The listing builds one solid part. Answer for the finished solid, in the listing's coordinates (mm). Coordinates: 2 decimals unless noted, no trailing zeros. Write each loop counter-clockwise with the first axis right and the second up, starting at its lowest first coordinate (ties: lowest second). Pieces come first, ordered by that corner, then holes.
(1) For a pull along Y with two mould halves and no side action, classify faces 1 (the flat face through (0, -10, 0)), 2 (the flat face through (0, 21, 2)), 3 (the cylindrical face through (-17, 15.57, 1.97)) as +Y half, -Y half, draft (parallel to the pull), parting line (faces both ways), or undercut.
(2) The part is cut by section C-C on x = 15.5. Determine the outline of the cut face in (y, z), plus the area to 3 significant figures.
(3) Straight lines are drawn through the part: line 1 (Y direction, x = -15.5, z = 2.85); line 2 (Y direction, x = 11, z = 1.2); line 3 (X direction, y = -32, z = 0.7). For each, find the intervals that lie inside material, in ascending order.
(4) The part is cut by section D-D on y = 0. Determine the outline of the cut face in (x, z), plus the area to 3 significant figures.
(5) The part is cut by section B-B on x = 0. Determine the outline of the cut face in (y, z).
(6) The part is cut by section A-A on y = -31. Determine the outline of the cut face in (x, z), plus the area to 3 significant figures.
from build123d import *

# Parameters (mm, degrees)
SKETCH1_W           = 42
SKETCH1_H           = 42
SKETCH1_R           = 4
SKETCH1_R_2         = 1.5
BOSS_EXTRUDE1_DEPTH = 4
SKETCH3_W           = 42
SKETCH3_H           = 4
BOSS_EXTRUDE2_DEPTH = 20
SKETCH4_R           = 2.5
CUT_EXTRUDE2_DEPTH  = 20


with BuildPart() as part:
    # Sketch1 → Boss-Extrude1 (new body)
    with BuildSketch(Plane.XY):
        Rectangle(SKETCH1_W, SKETCH1_H)
        Circle(SKETCH1_R, mode=Mode.SUBTRACT)
        with Locations((-15.5, 15.5)):
            Circle(SKETCH1_R_2, mode=Mode.SUBTRACT)
        with Locations((15.5, 15.5)):
            Circle(SKETCH1_R_2, mode=Mode.SUBTRACT)
        with Locations((15.5, -15.5)):
            Circle(SKETCH1_R_2, mode=Mode.SUBTRACT)
        with Locations((-15.5, -15.5)):
            Circle(SKETCH1_R_2, mode=Mode.SUBTRACT)
    extrude(amount=BOSS_EXTRUDE1_DEPTH)

    # Sketch3 → Boss-Extrude2 (add)
    with BuildSketch(Plane.XZ.offset(21)):
        with Locations((0, 2)):
            Rectangle(SKETCH3_W, SKETCH3_H)
    extrude(amount=BOSS_EXTRUDE2_DEPTH)

    # Sketch4 → Cut-Extrude2 (cut)
    with BuildSketch(Plane(origin=(0, 0, 0), x_dir=(-1, 0, 0), z_dir=(0, 0, -1))):
        with Locations((-11, -31)):
            Circle(SKETCH4_R)
        with Locations((11, -31)):
            Circle(SKETCH4_R)
    extrude(amount=-CUT_EXTRUDE2_DEPTH, mode=Mode.SUBTRACT)


solid = part.part
Model answer:
1. face 1: draft
1. face 2: +Y half
1. face 3: undercut
2. outline: (-41, 0) - (-17, 0) - (-17, 4) - (-41, 4) - close; (-14, 0) - (14, 0) - (14, 4) - (-14, 4) - close; (17, 0) - (21, 0) - (21, 4) - (17, 4) - close
2. area: 224 mm2
3. line 1: y = -41 to -17, -14 to 14, 17 to 21
3. line 2: y = -41 to -33.5, -28.5 to 21
3. line 3: x = -21 to -13.29, -8.71 to 8.71, 13.29 to 21
4. outline: (-21, 0) - (-4, 0) - (-4, 4) - (-21, 4) - close; (4, 0) - (21, 0) - (21, 4) - (4, 4) - close
4. area: 136 mm2
5. outline: (-41, 0) - (-4, 0) - (-4, 4) - (-41, 4) - close; (4, 0) - (21, 0) - (21, 4) - (4, 4) - close
6. outline: (-21, 0) - (-13.5, 0) - (-13.5, 4) - (-21, 4) - close; (-8.5, 0) - (8.5, 0) - (8.5, 4) - (-8.5, 4) - close; (13.5, 0) - (21, 0) - (21, 4) - (13.5, 4) - close
6. area: 128 mm2
